from build123d import *

# Parameters (mm, degrees)
SKETCH1_W           = 66
SKETCH1_H           = 66
SKETCH1_W_2         = 60
SKETCH1_H_2         = 60
EXTRUDE_THIN1_DEPTH = 15
BOSS_EXTRUDE1_START = 15
SKETCH1_2_W         = 60
SKETCH1_2_H         = 60
BOSS_EXTRUDE1_DEPTH = 5
SKETCH2_R           = 1.55
CUT_EXTRUDE1_DEPTH  = 50.020403915
SKETCH2_2_R         = 3.55
SKETCH2_2_R_2       = 1.55
EXTRUDE_THIN2_DEPTH = 15
SKETCH3_R           = 11.9
SKETCH3_R_2         = 7.9
BOSS_EXTRUDE2_DEPTH = 6


with BuildPart() as part:
    # Sketch1 → Extrude-Thin1 (new body)
    with BuildSketch(Plane.XY):
        Rectangle(SKETCH1_W, SKETCH1_H)
        Rectangle(SKETCH1_W_2, SKETCH1_H_2, mode=Mode.SUBTRACT)
    extrude(amount=EXTRUDE_THIN1_DEPTH)

    # Sketch1<2> → Boss-Extrude1 (add)
    with BuildSketch(Plane.XY.offset(BOSS_EXTRUDE1_START)):
        Rectangle(SKETCH1_2_W, SKETCH1_2_H)
    extrude(amount=-BOSS_EXTRUDE1_DEPTH)

    # Sketch2 → Cut-Extrude1 (cut, through all)
    with BuildSketch(Plane.XY.offset(15)):
        with Locations((22.384300197, 22.867949289)):
            Circle(SKETCH2_R)
        with Locations((22.867949289, -22.384300197)):
            Circle(SKETCH2_R)
        with Locations((-22.384300197, -22.867949289)):
            Circle(SKETCH2_R)
        with Locations((-22.867949289, 22.384300197)):
            Circle(SKETCH2_R)
    extrude(amount=-CUT_EXTRUDE1_DEPTH, mode=Mode.SUBTRACT)

    # Sketch2<2> → Extrude-Thin2 (add)
    # profile 1 of 4: a face of its own
    with BuildSketch(Plane.XY.offset(15)):
        with Locations((22.384300197, 22.867949289)):
            Circle(SKETCH2_2_R)
        with Locations((22.384300197, 22.867949289)):
            Circle(SKETCH2_2_R_2, mode=Mode.SUBTRACT)
    # profile 2 of 4: a face of its own
    with BuildSketch(Plane.XY.offset(15)):
        with Locations((22.867949289, -22.384300197)):
            Circle(SKETCH2_2_R)
        with Locations((22.867949289, -22.384300197)):
            Circle(SKETCH2_2_R_2, mode=Mode.SUBTRACT)
    # profile 3 of 4: a face of its own
    with BuildSketch(Plane.XY.offset(15)):
        with Locations((-22.384300197, -22.867949289)):
            Circle(SKETCH2_2_R)
        with Locations((-22.384300197, -22.867949289)):
            Circle(SKETCH2_2_R_2, mode=Mode.SUBTRACT)
    # profile 4 of 4: a face of its own
    with BuildSketch(Plane.XY.offset(15)):
        with Locations((-22.867949289, 22.384300197)):
            Circle(SKETCH2_2_R)
        with Locations((-22.867949289, 22.384300197)):
            Circle(SKETCH2_2_R_2, mode=Mode.SUBTRACT)
    extrude(amount=-EXTRUDE_THIN2_DEPTH)

    # Sketch3 → Boss-Extrude2 (add)
    with BuildSketch(Plane.XY.offset(15)):
        Circle(SKETCH3_R)
        Circle(SKETCH3_R_2, mode=Mode.SUBTRACT)
    extrude(amount=BOSS_EXTRUDE2_DEPTH)


solid = part.part
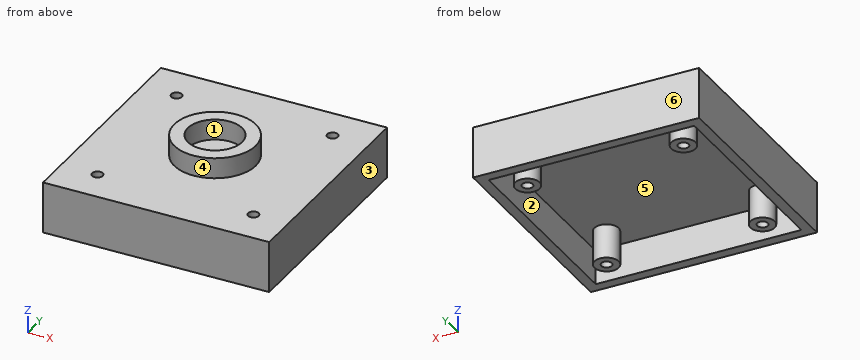
Can you work these out from the model? Positions are in its coordinate system, mm. Face numbers are marked on the shaded views. A direction names the side the tool comes from. Coordinates: 2 decimals unless noted, no trailing zeros. Write each loop counter-clockwise with the first axis right and the second up, starting at its lowest first coordinate (ties: lowest second). Pieces come first, ordered by that corner, then holes. Notation, with made-up numbers: (19, 88) -> (56, 88) arc R12 cw to (56, 110) -> close; hole circle Ø10 at (-19.5, -20.5). An arc over 180 degrees is marked (long way). Answer as CSV lines item,"result".
1) Will these pins go through, and if not, where does the flat tip stop? P1, Ø12.5, axis at x = 0, y = 0, coming from the -Z side; P2, Ø12, axis at x = 23, y = -5.5, coming from the +Z side.
Check result:
P1,"z = 10"
P2,"z = 15"
2) If we mould it in two halves opening along X, with no side actions, what happens to the marked faces 4, 5 and 6? For each: +X half, -X half, draft (parallel to the pull), parting line (faces both ways), or undercut.
Check result:
face 4,"parting line"
face 5,"undercut"
face 6,"draft"
3) If I drill on line 1 (Y direction, x = 0, z = 16.6); line 2 (X direction, y = 29.5, z = 3.25), over which ranges is the centre line in solid material (lowest first)? Write a range as from..to.
Check result:
line 1,"-11.9..-7.9, 7.9..11.9"
line 2,"-33..-30, 30..33"
4) If we section it at A-A on x = -15: Please give me the cut outline in (y, z), then the cut area to 3 significant figures.
Check result:
outline,"(-33, 0) -> (-30, 0) -> (-30, 10) -> (30, 10) -> (30, 0) -> (33, 0) -> (33, 15) -> (-33, 15) -> close"
area,"390 mm²"
5) If we section it at D-D on z = 7.75: Count the separate pieces of the cut face and the enclosed holes in it, then the cut area to 3 significant figures.
Check result:
separate pieces,"5"
enclosed holes,"5"
area,"884 mm²"
6) On a 3-axis mill with a long thin cutter (end or side, diameter ignored), from which of +Z, -Z, +X, -X, +Y, -Y can I reach the whole of each face in a straight line? I mean the marked faces 1, 2 and 3. Say none if no direction works.
Check result:
face 1,"+Z"
face 2,"-Z"
face 3,"+Z, -Z, +X, +Y, -Y"
7) If we section it at B-B on y = 0: Please give me the cut outline in (x, z).
Check result:
outline,"(-33, 0) -> (-30, 0) -> (-30, 10) -> (30, 10) -> (30, 0) -> (33, 0) -> (33, 15) -> (11.9, 15) -> (11.9, 21) -> (7.9, 21) -> (7.9, 15) -> (-7.9, 15) -> (-7.9, 21) -> (-11.9, 21) -> (-11.9, 15) -> (-33, 15) -> close"
8) If we section it at C-C on x = 23: Please give me the cut outline in (y, z).
Check result:
outline,"(-33, 0) -> (-30, 0) -> (-30, 10) -> (-25.93, 10) -> (-25.93, 0) -> (-23.93, 0) -> (-23.93, 15) -> (-33, 15) -> close; (-20.84, 0) -> (-18.84, 0) -> (-18.84, 10) -> (19.37, 10) -> (19.37, 0) -> (21.45, 0) -> (21.45, 15) -> (-20.84, 15) -> close; (24.29, 0) -> (26.36, 0) -> (26.36, 10) -> (30, 10) -> (30, 0) -> (33, 0) -> (33, 15) -> (24.29, 15) -> close"
